```python
from build123d import *

# Parameters (mm, degrees)
F1_R      = 56.692647
F2_DEPTH  = 25.4
F3_R      = 37.015335
F4_DEPTH  = 25.4
F4_FACE_R = 37.015335
F5_DEPTH  = 25.4
F6_R      = 26.874767
F7_DEPTH  = 25.4


with BuildPart() as f2:
    # F1 (on face) → F2 (new body)
    with BuildSketch(Plane.XZ):
        with Locations((0, 18.79701)):
            Circle(F1_R)
    extrude(amount=F2_DEPTH)

    # F3 (on face) → F4 (join)
    with BuildSketch(Plane.XZ.offset(25.4)):
        with Locations((-37.807173, 61.042411)):
            Circle(F3_R)
    extrude(amount=F4_DEPTH)

    # F4_face (on face) → F5 (join)
    with BuildSketch(Plane(origin=(-37.807173, -50.8, 61.042411), x_dir=(1, 0, 0), z_dir=(0, -1, 0))):
        Circle(F4_FACE_R)
    extrude(amount=F5_DEPTH)

    # F6 (on face) → F7 (join)
    with BuildSketch(Plane.XZ):
        with Locations((0, 20.070814)):
            Circle(F6_R)
    extrude(amount=F7_DEPTH)


solid = f2.part
```
For this review, take the finished solid that the model builds, in its own axes (mm). A direction names the side the tool comes from. Give positions to 0.01 mm unless a question says otherwise; leave off trailing zeros. Write each loop counter-clockwise with the first axis right and the second up, starting at its lowest first coordinate (ties: lowest second). Pieces come first, ordered by that corner, then holes. Notation, with made-up numbers: M 61.5,64.25 L 66.5,64.25 A11 cw 66.5,73.25 Z; hole C 57,1 d5. An arc over 180 degrees is marked long. Answer as a JSON object with one key per item and string values. Group by question number.
Item 1: Consider section B-B on x = 48. Write out the cut boundary in (y, z).
Item 2: Consider section C-C on y = -22.5. Write out the cut boundary in (x, z), plus the area to 3 significant figures.
Item 3: Tool access review of faces 1 (the flat face through (-48, -25.4, 72)), 2 (the cylindrical face through (-2.5, -50.44, 72.16)), 3 (the flat face through (-1, 0, 20)), 4 (the flat face through (-38, -76.2, 62)), 5 (the cylindrical face through (-12.29, -12.522, -36.548)): name each direction out of +Z, -Z, +X, -X, +Y, -Y from which nothing blocks a thin tool from reaching the whole face with its end or side.
Item 4: Consider section A-A on z = 67. Write out the cut boundary in (x, y), plus the area to 3 significant figures.
Item 5: Consider section D-D on z = 44.5. Write out the cut boundary in (x, y).
Item 6: For pin 1 Ø5 at (x, y) = (34.5, -24) entering from -Z; pin 2 Ø1.5 at (y, z) = (-22, 28.5) entering from -X; pin 3 Ø10 at (x, z) = (15.5, 36) entering from -Y, all flat-tipped, find the tip position at first contact; note any pin that passes through.
Item 7: For probe 1 along Y at (x, z) = (51, 3); probe 2 along Y at (x, z) = (-52, 42); probe 3 along X at (y, z) = (-29.5, 62.5), list the stretches that pass through material, from the lowest coordinate up. Write a range as [from, to].
Check result:
{
 "1": {"outline": "M -25.4,-11.37 L 0,-11.37 L 0,48.96 L -25.4,48.96 Z"},
 "2": {"outline": "C 0,18.8 d113.39", "area": "10,100 mm^2"},
 "3": {"face 1": "+Z, -X, +Y", "face 2": "-Y", "face 3": "+Z, -Z, +X, -X, +Y", "face 4": "+Z, -Z, +X, -X, -Y", "face 5": "+Y"},
 "4": {"outline": "M -74.34,-76.2 L -1.27,-76.2 L -1.27,-25.4 L 29.84,-25.4 L 29.84,0 L -29.84,0 L -29.84,-25.4 L -74.34,-25.4 Z", "area": "5,230 mm^2"},
 "5": {"outline": "M -70.92,-76.2 L -4.69,-76.2 L -4.69,-25.4 L 50.53,-25.4 L 50.53,0 L -50.53,0 L -50.53,-25.4 L -70.92,-25.4 Z"},
 "6": {"pin 1": "stops at z = -28", "pin 2": "stops at x = -55.98", "pin 3": "stops at y = -25.4"},
 "7": {"probe 1": "y = [-25.4, 0]", "probe 2": "y = [-76.2, -25.4]", "probe 3": "x = [-74.79, -0.82]"}
}
